Geometry: final body of the model. Coordinates: model frame, mm. A direction names the side the tool comes from. Round coordinates to 2 decimals unless told otherwise and drop trailing zeros. Order: outer loops, then holes, each group sorted by start corner. A loop starts at its lowest first (then second) coordinate and runs counter-clockwise, first axis right, second up. Notation, with made-up numbers: M 36.5,66 L 89.5,66 A20 ccw 89.5,94 Z; hole C -18,73 d5. An arc over 180 degrees is marked long. Put each result on its own line as item: value. Start each with the question number.
1) Access query for faces 1 (the cylindrical face through (-0.29, -2.23, -0.49)), 2 (the flat face through (2, -2, 0)). Directions: +Z, -Z, +X, -X, +Y, -Y. A direction counts if a zero-diameter tool reaches every point of the face in a straight line with its end or side. Return the directions, or none.
2) Section D-D, the plane x = -3.25. Return loops of the section in (y, z).
3) Material intervals for probe 1 along Y at (x, z) = (0, -0.25); probe 2 along Y at (x, z) = (-0.5, 2.25); probe 3 along Z at (x, y) = (-2.75, 0.5), sorted ascending. Write a range as [from, to].
4) First-contact query: P1, Ø1, axis at x = 1, y = 1, coming from the +Z side; P2, Ø2, axis at y = -3, z = 3, coming from the -X side; P3, Ø1.5, axis at y = 1, z = 2.5, coming from the -X side. Flat tips, straight axial feed; report the tip coordinate or a pass-through.
5) Section A-A, the plane z = 0.35. Return loops of the section in (x, y), then the cut area to 3 significant figures.
6) Section B-B, the plane x = 0. Return loops of the section in (y, z), then the cut area to 3 significant figures.
7) Section C-C, the plane y = 2. Return loops of the section in (x, z).
8) Draft query along Y for faces 3 (the flat face through (0, 4.3, 1)), 4 (the flat face through (3.09, -1.75, 1.73)), 5 (the flat face through (3.74, -2.12, 1.28)), 6 (the flat face through (-3.09, 1.75, 1.73)). Return one class per face: pulls with the +Y half, pulls with the -Y half, needs draft (parallel to the pull), parting line crosses it, or undercut.
from build123d import *

# Parameters (mm, degrees)
F1_DEPTH = 3.5
F2_R     = 2.25
F3_DEPTH = 1


with BuildPart() as f1:
    # F0 (on Top) → F1 (new body)
    with BuildSketch(Plane.XY):
        Polygon((-2.482606, -4.3), (2.482606, -4.3), (4.965212, 0), (2.482606, 4.3), (-2.482606, 4.3), (-4.965212, 0), align=None)
        Polygon((4.099187, 0), (2.049593, -3.55), (-2.049593, -3.55), (-4.099187, 0), (-2.049593, 3.55), (2.049593, 3.55), align=None, mode=Mode.SUBTRACT)
    extrude(amount=F1_DEPTH)

    # F2 (on face) → F3 (join)
    with BuildSketch(Plane(origin=(0, 0, 0), x_dir=(1, 0, 0), z_dir=(0, 0, -1))):
        Polygon((4.965212, 0), (2.482606, 4.3), (-2.482606, 4.3), (-4.965212, 0), (-2.482606, -4.3), (2.482606, -4.3), align=None)
        Circle(F2_R, mode=Mode.SUBTRACT)
    extrude(amount=F3_DEPTH)


solid = f1.part
Result sheet:
1. face 1: +Z, -Z
1. face 2: +Z
2. outline: M -2.97,-1 L 2.97,-1 L 2.97,3.5 L 1.47,3.5 L 1.47,0 L -1.47,0 L -1.47,3.5 L -2.97,3.5 Z
3. probe 1: y = [-4.3, -2.25], [2.25, 4.3]
3. probe 2: y = [-4.3, -3.55], [3.55, 4.3]
3. probe 3: z = [-1, 0]
4. P1: passes through
4. P2: stops at x = -3.81
4. P3: stops at x = -4.82
5. outline: M -4.97,0 L -2.48,-4.3 L 2.48,-4.3 L 4.97,0 L 2.48,4.3 L -2.48,4.3 Z; hole M -4.1,0 L -2.05,-3.55 L 2.05,-3.55 L 4.1,0 L 2.05,3.55 L -2.05,3.55 Z
5. area: 20.4 mm2
6. outline: M -4.3,-1 L -2.25,-1 L -2.25,0 L -3.55,0 L -3.55,3.5 L -4.3,3.5 Z; M 2.25,-1 L 4.3,-1 L 4.3,3.5 L 3.55,3.5 L 3.55,0 L 2.25,0 Z
6. area: 9.35 mm2
7. outline: M -3.81,-1 L -1.03,-1 L -1.03,0 L -2.94,0 L -2.94,3.5 L -3.81,3.5 Z; M 1.03,-1 L 3.81,-1 L 3.81,3.5 L 2.94,3.5 L 2.94,0 L 1.03,0 Z
8. face 3: pulls with the +Y half
8. face 4: undercut
8. face 5: pulls with the -Y half
8. face 6: undercut
